Can you work these out from the model? Positions are in its coordinate system, mm. Face numbers are marked on the shaded views. Coordinates: 2 decimals unless noted, no trailing zeros. Loops run counter-clockwise (first coordinate to the right, second up) from the corner with the lowest first, then second, coordinate; pieces in that order, holes last. Notation, with made-up numbers: M 72.5,50.5 L 89.5,50.5 A22 cw 89.5,64.5 Z; hole C -36.75,49.5 d2. An arc over 180 degrees is marked long. Return JSON: item names as keys, results as strings. Group by question number.
```python
from build123d import *

# Parameters (mm, degrees)
SKETCH1_R               = 25
SKETCH1_R_2             = 22.5
BOSS_EXTRUDE1_DEPTH     = 194
CUT_EXTRUDE1_DEPTH      = 198.19533463
CUT_EXTRUDE1_DEPTH_BACK = 198.19533463
SKETCH10_R              = 2


with BuildPart() as part:
    # Sketch1 → Boss-Extrude1 (new body)
    with BuildSketch(Plane.XY):
        Circle(SKETCH1_R)
        Circle(SKETCH1_R_2, mode=Mode.SUBTRACT)
    extrude(amount=-BOSS_EXTRUDE1_DEPTH)

    # Sketch10 → Cut-Extrude1 (cut, two sides: drawn at the far end of the back side and taken through both)
    with BuildSketch(Plane(origin=(0, 0, 0), x_dir=(1, 0, 0), z_dir=(0, 1, 0)).offset(-CUT_EXTRUDE1_DEPTH_BACK)):
        with Locations(Location((0, 156, 0), (0, 0, 270))):
            Circle(SKETCH10_R)
        with Locations(Location((0, 19, 0), (0, 0, 270))):
            Circle(SKETCH10_R)
    extrude(amount=CUT_EXTRUDE1_DEPTH + CUT_EXTRUDE1_DEPTH_BACK, mode=Mode.SUBTRACT)


solid = part.part
```
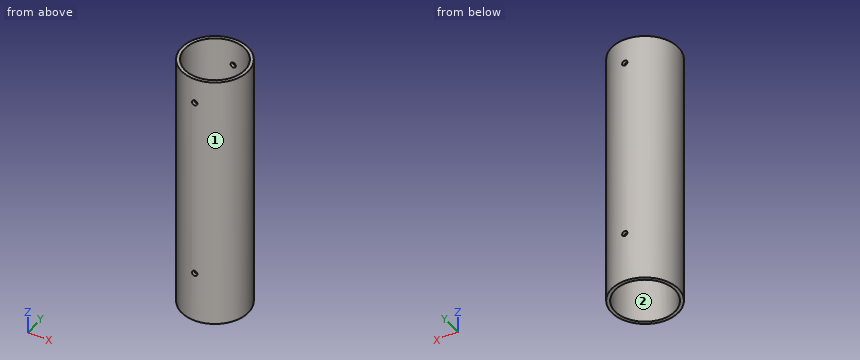
1) If we mould it in two halves opening along X, with no side actions, what happens to the marked faces 1 and 2? For each: +X half, -X half, draft (parallel to the pull), parting line (faces both ways), or undercut.
2) If I drill on line 1 (Z direction, x = 0, y = -23.65); line 2 (Y direction, x = 15, z = -9); line 3 (X direction, y = 23, z = -156), over which ranges is the centre line in solid material (lowest first)? Write a range as from..to.
3) Suppose I cut it at B-B, the plane y = 2.5. List the corners of the cut face in (x, z) for me, then the cut area to 3 significant figures.
4) Suppose I cut it at C-C, the plane z = -156. List the corners of the cut face in (x, y) for me, then the cut area to 3 significant figures.
5) Suppose I cut it at A-A, the plane x = 0. List the corners of the cut face in (y, z) for me.
6) For pin 1 (2.5 mm diameter, centred on x = 0, z = -19, fed in from +Y); pin 2 (12 mm diameter, centred on x = -19, z = -154.5, fed in from -Y); pin 3 (10 mm diameter, centred on y = -10, z = -69.5, fed in from +X); pin 4 (1.5 mm diameter, centred on x = -5.5, z = -153.5, fed in from -Y), each with a flat end and sliding along its axis, tell me the tip position at first contact or that it passes through.
7) Suppose I cut it at D-D, the plane z = -27. List the corners of the cut face in (x, y) for me.
Returned:
{
 "1": {"face 1": "parting line", "face 2": "undercut"},
 "2": {"line 1": "z = -194..-158, -154..-21, -17..0", "line 2": "y = -20..-16.77, 16.77..20", "line 3": "x = -9.8..-2, 2..9.8"},
 "3": {"outline": "M -24.87,-194 L -22.36,-194 L -22.36,0 L -24.87,0 Z; M 22.36,-194 L 24.87,-194 L 24.87,0 L 22.36,0 Z", "area": "975 mm²"},
 "4": {"outline": "M -2,-24.92 L -2,-22.41 A22.5 cw -2,22.41 L -2,24.92 A25 ccw Z; M 2,-24.92 A25 ccw 2,24.92 L 2,22.41 A22.5 cw 2,-22.41 Z", "area": "353 mm²"},
 "5": {"outline": "M -25,-194 L -22.5,-194 L -22.5,-158 L -25,-158 Z; M -25,-154 L -22.5,-154 L -22.5,-21 L -25,-21 Z; M -25,-17 L -22.5,-17 L -22.5,0 L -25,0 Z; M 22.5,-194 L 25,-194 L 25,-158 L 22.5,-158 Z; M 22.5,-154 L 25,-154 L 25,-21 L 22.5,-21 Z; M 22.5,-17 L 25,-17 L 25,0 L 22.5,0 Z"},
 "6": {"pin 1": "passes through", "pin 2": "stops at y = -21.35", "pin 3": "stops at x = 24.49", "pin 4": "stops at y = -24.54"},
 "7": {"outline": "C 0,0 d50; hole C 0,0 d45"}
}
